from build123d import *

# Parameters (mm, degrees)
F1_DEPTH = 152.4
F2_W     = 101.6
F2_H     = 76.2
F3_DEPTH = 76.2
F5_DEPTH = 76.2
F7_D     = 12.7
F9_D     = 9.525


with BuildPart() as f1:
    # F0 (on Front) → F1 (new body)
    with BuildSketch(Plane.XZ):
        Polygon((0, 152.4), (-50.8, 152.4), (-50.8, -50.8), (101.6, -50.8), (101.6, 0), (0, 0), align=None)
    extrude(amount=F1_DEPTH)

    # F2 (on face) → F3 (join)
    with BuildSketch(Plane.XY):
        with Locations((50.8, -38.1)):
            Rectangle(F2_W, F2_H)
    extrude(amount=F3_DEPTH)

    # F4 (on face) → F5 (cut)
    with BuildSketch(Plane.XZ.offset(76.2)):
        Polygon((101.6, 76.2), (0, 76.2), (101.6, 0), align=None)
    extrude(amount=-F5_DEPTH, mode=Mode.SUBTRACT)

    # F7 (through all)
    with Locations(Plane.YZ):
        with Locations((-114.3, 114.3)):
            Hole(F7_D / 2)

    # F9 (through all)
    with Locations(Plane.XY):
        with Locations((63.5, -114.3)):
            Hole(F9_D / 2)


solid = f1.part
Input: part model. Units: mm. Frame: model coordinates. A direction names the side the tool comes from. Round coordinates to 2 decimals unless told otherwise and drop trailing zeros. Order: outer loops, then holes, each group sorted by start corner. A loop starts at its lowest first (then second) coordinate and runs counter-clockwise, first axis right, second up. Notation, with made-up numbers: (33.5, 20) - (48.5, 20) arc R12 cw to (48.5, 27) - close; hole circle Ø11 at (32.5, -31.5). An arc over 180 degrees is marked (long way). Use a Markdown table: item, result.
1. Mould query, pull axis X, two halves, no side actions, for faces 3 (the face through (0, -92, 92)), 4 (the face through (-10, -152.4, 30)), 5 (the face through (67.28, -117.2, -25.76)). Classes: +X half, -X half, draft (parallel to the pull), parting line (faces both ways), or undercut.
Evaluation:
| item | result |
|---|---|
| face 3 | +X half |
| face 4 | draft |
| face 5 | undercut |
2. Section D-D on y = -67. Return the cut outline in (x, z), then the cut area to 3 significant figures.
Evaluation:
| item | result |
|---|---|
| outline | (-50.8, -50.8) - (101.6, -50.8) - (101.6, 0) - (0, 76.2) - (0, 152.4) - (-50.8, 152.4) - close |
| area | 19,400 mm^2 |
3. First-contact query: pin 1 (3 mm diameter, centred on y = -113.5, z = 29, fed in from +X); pin 2 (8.5 mm diameter, centred on x = 63.5, y = -114.3, fed in from -Z); pin 3 (3 mm diameter, centred on x = 27, y = -79, fed in from +Z). Flat tips, straight axial feed; report the tip coordinate or a pass-through.
Evaluation:
| item | result |
|---|---|
| pin 1 | x = 0 |
| pin 2 | through |
| pin 3 | z = 0 |
4. Access query for faces 1 (the face through (-25, -75, 152.4)), 2 (the face through (52, -114, 0)). Directions: +Z, -Z, +X, -X, +Y, -Y. A direction counts if a zero-diameter tool reaches every point of the face in a straight line with its end or side. Return the directions, or none.
Evaluation:
| item | result |
|---|---|
| face 1 | +Z, +X, -X, +Y, -Y |
| face 2 | +Z, +X, -Y |
5. Section A-A on y = -114.3. Return the cut outline in (x, z).
Evaluation:
| item | result |
|---|---|
| outline | (-50.8, -50.8) - (58.74, -50.8) - (58.74, 0) - (0, 0) - (0, 107.95) - (-50.8, 107.95) - close; (-50.8, 120.65) - (0, 120.65) - (0, 152.4) - (-50.8, 152.4) - close; (68.26, -50.8) - (101.6, -50.8) - (101.6, 0) - (68.26, 0) - close |
6. Section C-C on x = 76. Return the cut outline in (y, z).
Evaluation:
| item | result |
|---|---|
| outline | (-152.4, -50.8) - (0, -50.8) - (0, 19.2) - (-76.2, 19.2) - (-76.2, 0) - (-152.4, 0) - close |
7. Material intervals for probe 1 along Y at (x, z) = (63.5, -36.5); probe 2 along Z at (x, y) = (-30, -114); probe 3 along X at (y, z) = (-43, 135), sorted ascending.
Evaluation:
| item | result |
|---|---|
| probe 1 | -152.4 to -119.06, -109.54 to 0 |
| probe 2 | -50.8 to 107.96, 120.64 to 152.4 |
| probe 3 | -50.8 to 0 |
8. Section B-B on z = 114.3. Return the cut outline in (x, y).
Evaluation:
| item | result |
|---|---|
| outline | (-50.8, -152.4) - (0, -152.4) - (0, -120.65) - (-50.8, -120.65) - close; (-50.8, -107.95) - (0, -107.95) - (0, 0) - (-50.8, 0) - close |
